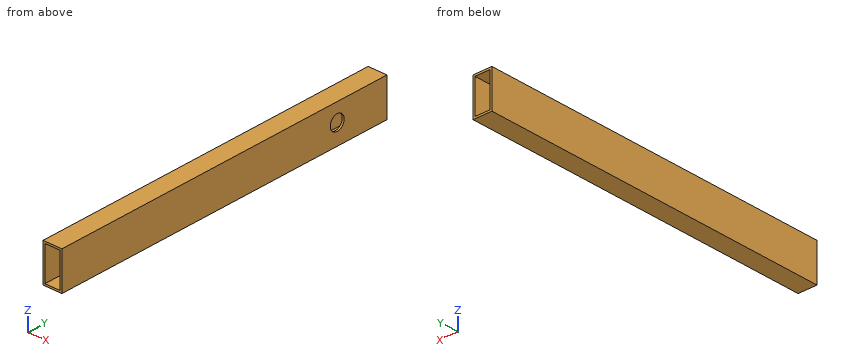
```python
from build123d import *

# Parameters (mm, degrees)
F0_W     = 20
F0_H     = 40
F0_W_2   = 16
F0_H_2   = 36
F1_DEPTH = 375
F2_R     = 8
F3_DEPTH = 15


with BuildPart() as f1:
    # F0 (on Front) → F1 (new body)
    with BuildSketch(Plane.XZ):
        with Locations((10, -20)):
            Rectangle(F0_W, F0_H)
        with Locations((10, -20)):
            Rectangle(F0_W_2, F0_H_2, mode=Mode.SUBTRACT)
    extrude(amount=F1_DEPTH)

    # F2 (on face) → F3 (cut)
    with BuildSketch(Plane.YZ.offset(20)):
        with Locations((-57.451189, -18.785227)):
            Circle(F2_R)
    extrude(amount=-F3_DEPTH, mode=Mode.SUBTRACT)


solid = f1.part
```
CAD build for the part. Positions are in the model's coordinates, mm. Give positions to 0.01 mm unless a question says otherwise; leave off trailing zeros. Order: outer loops, then holes, each group sorted by start corner. A loop starts at its lowest first (then second) coordinate and runs counter-clockwise, first axis right, second up.
(1) Saw through at C-C, the plane y = -36.5. Give the cut face in (x, z).
(2) Saw through at A-A, the plane x = 6.75. Give the cut face in (y, z), then the cut area to 3 significant figures.
(3) Flat gauge pin, fed straight in: pin 1 (8 mm diameter, centred on x = 13, z = -12, fed in from -Y). Where does the tip first touch, or does it go through?
(4) Saw through at B-B, the plane z = -32. Give the cut face in (x, y).
(5) Drill centre lines: L1, parallel to X at y = -164, z = -18; L2, parallel to Z at x = 6.5, y = -102.5; L3, parallel to Y at x = 18.5, z = -14.5. Where is each one in solid material? Low to high.
Results found:
1. outline: (0, -40) - (20, -40) - (20, 0) - (0, 0) - close; hole (2, -38) - (18, -38) - (18, -2) - (2, -2) - close
2. outline: (-375, -40) - (0, -40) - (0, -38) - (-375, -38) - close; (-375, -2) - (0, -2) - (0, 0) - (-375, 0) - close
2. area: 1,500 mm2
3. pin 1: passes through
4. outline: (0, -375) - (2, -375) - (2, 0) - (0, 0) - close; (18, -375) - (20, -375) - (20, 0) - (18, 0) - close
5. L1: x = 0 to 2, 18 to 20
5. L2: z = -40 to -38, -2 to 0
5. L3: y = -375 to -64.21, -50.7 to 0
